from build123d import *

# Parameters (mm, degrees)
SKETCH_1_R                = 31
EXTRUDE_1_DEPTH           = 10
HOLE_WIZARD_M5_2_D        = 4.2
HOLE_WIZARD_2_D           = 4.5
HOLE_WIZARD_2_CBORE_D     = 8
HOLE_WIZARD_2_CBORE_DEPTH = 4.6


with BuildPart() as part:
    # 草图1 → 凸台-拉伸1 (new body)
    with BuildSketch(Plane(origin=(0, 0, 0), x_dir=(1, 0, 0), z_dir=(0, 1, 0))):
        with Locations(Location((0, 0, 0), (0, 0, 270))):
            Circle(SKETCH_1_R)
    extrude(amount=EXTRUDE_1_DEPTH)

    # M5 螺纹孔2 (through all)
    with Locations(Plane(origin=(-21, 10, 0), x_dir=(0, 0, 1), z_dir=(0, 1, 0))):
        with Locations((0, 0), (0, 42)):
            Hole(HOLE_WIZARD_M5_2_D / 2)

    # 打孔尺寸(%根据)内六角圆柱头螺钉的类型2 (through all)
    with Locations(Plane(origin=(-11.136931804, 0, 11.136931804), x_dir=(0, 0, -1), z_dir=(0, -1, 0))):
        with Locations((0, 0), (0, 22.273863608), (22.273863608, 22.273863608), (22.273863608, 0)):
            CounterBoreHole(HOLE_WIZARD_2_D / 2, HOLE_WIZARD_2_CBORE_D / 2, HOLE_WIZARD_2_CBORE_DEPTH)


solid = part.part
CAD build for the part. Positions are in the model's coordinates, mm. A direction names the side the tool comes from. Coordinates: 2 decimals unless noted, no trailing zeros. Write each loop counter-clockwise with the first axis right and the second up, starting at its lowest first coordinate (ties: lowest second). Pieces come first, ordered by that corner, then holes. Notation, with made-up numbers: (25.25, 76.25) - (34.25, 76.25) arc R23 ccw to (34.25, 88.25) - close; hole circle Ø7 at (69.25, 89). An arc over 180 degrees is marked (long way). Use a Markdown table: item, result. Add a question column.
Item 1: Band-saw the part on B-B, the plane x = -12.5. Give the cut face in (y, z).
Item 2: Band-saw the part on D-D, the plane y = 2. Give the cut face in (x, z).
Item 3: Drill centre lines: L1, parallel to X at y = 6.5, z = 0; L2, parallel to X at y = 7.5, z = -11; L3, parallel to Y at x = 15, z = -11.5. Where is each one in solid material? Low to high. Write a range as from..to.
Item 4: Band-saw the part on C-C, the plane x = -21. Give the cut face in (y, z), and give its area (3 significant figures).
Item 5: Band-saw the part on A-A, the plane z = 0. Give the cut face in (x, y), and give its area (3 significant figures).
Item 6: Flat gauge pins, fed straight in: pin 1 (1.5 mm diameter, centred on x = -4.5, y = 5, fed in from -Z); pin 2 (4 mm diameter, centred on x = 10, z = 10.5, fed in from -Y); pin 3 (3 mm diameter, centred on y = 4.5, z = -14.5, fed in from +X). Where does each tip first touch, or does it go through?
Item 7: 3-axis set-ups, long thin cutter, end or side, ignore diameter. For faces 1 (the face through (9.14, 7.34, -10.1)), 2 (the face through (-13, 4.6, 9)): which of +Z, -Z, +X, -X, +Y, -Y reach the whole face in a straight line?
Numbers:
| question | item | result |
|---|---|---|
| 1 | outline | (0, -28.37) - (10, -28.37) - (10, -12.93) - (4.6, -12.93) - (4.6, -14.9) - (0, -14.9) - close; (0, -7.38) - (4.6, -7.38) - (4.6, -9.35) - (10, -9.35) - (10, 9.35) - (4.6, 9.35) - (4.6, 7.38) - (0, 7.38) - close; (0, 14.9) - (4.6, 14.9) - (4.6, 12.93) - (10, 12.93) - (10, 28.37) - (0, 28.37) - close |
| 2 | outline | circle Ø62 at (0, 0); hole circle Ø4.2 at (-21, 0); hole circle Ø8 at (-11.14, -11.14); hole circle Ø8 at (-11.14, 11.14); hole circle Ø8 at (11.14, -11.14); hole circle Ø8 at (11.14, 11.14); hole circle Ø4.2 at (21, 0) |
| 3 | L1 | -31..-23.1, -18.9..18.9, 23.1..31 |
| 3 | L2 | -28.98..-13.38, -8.89..8.89, 13.38..28.98 |
| 3 | L3 | 4.6..10 |
| 4 | outline | (0, -22.8) - (10, -22.8) - (10, -2.1) - (0, -2.1) - close; (0, 2.1) - (10, 2.1) - (10, 22.8) - (0, 22.8) - close |
| 4 | area | 414 mm2 |
| 5 | outline | (-31, 0) - (-23.1, 0) - (-23.1, 10) - (-31, 10) - close; (-18.9, 0) - (18.9, 0) - (18.9, 10) - (-18.9, 10) - close; (23.1, 0) - (31, 0) - (31, 10) - (23.1, 10) - close |
| 5 | area | 536 mm2 |
| 6 | pin 1 | z = -30.77 |
| 6 | pin 2 | y = 4.6 |
| 6 | pin 3 | x = 28.14 |
| 7 | face 1 | +Y, -Y |
| 7 | face 2 | -Y |
